Autodesk Inventor part; units mm, degrees
ref_plane "YZ Plane" through (0, 0, 0) normal (1, 0, 0) x (0, 1, 0)
ref_plane "XZ Plane" through (0, 0, 0) normal (0, 1, 0) x (-1, 0, 0)
ref_plane "XY Plane" through (0, 0, 0) normal (0, 0, 1) x (1, 0, 0)
sketch "Sketch1" plane through (0, 0, 0) normal (0, 1, 0) x (-1, 0, 0)
  line L0 (-5.5, -5.5) -> (-2, -5.5)
  line L1 (5.5, -0.5) -> (5.5, -0.5)
  line L2 (5.5, 5.5) -> (-5.5, 5.5)
  line L3 (-5.5, -0.5) -> (-5.5, -0.5)
  line L4 (-5.5, -5.5) -> (5.5, 5.5) construction
  line L5 (5.5, -5.5) -> (-5.5, 5.5) construction
  circle A0 centre (2.5, 2.5) radius 1
  circle A1 centre (-2.5, 2.5) radius 1
  line L6 (5.5, 5.5) -> (5.5, 2)
  line L7 (-5.5, 5.5) -> (-5.5, -5.5)
  circle A2 centre (-2.5, -2.5) radius 1
  arc A3 (-2, -5.5) -> (5.5, 2) centre (-2, 2) ccw
  point P0 (0, 0)
  dimension "d1" = 11
  dimension "d3" = 2
  dimension "d4" = 2
  dimension "d5" = 3
  dimension "d6" = 3
  dimension "d7" = 3
  dimension "d8" = 3
  dimension "d12" = 11
  dimension "d13" = 2
  dimension "d14" = 3
  dimension "d15" = 3
  dimension "d16" = 7.5
extrude "Extrusion1" add sketch "Sketch1" along normal blind 5
properties part number "link"
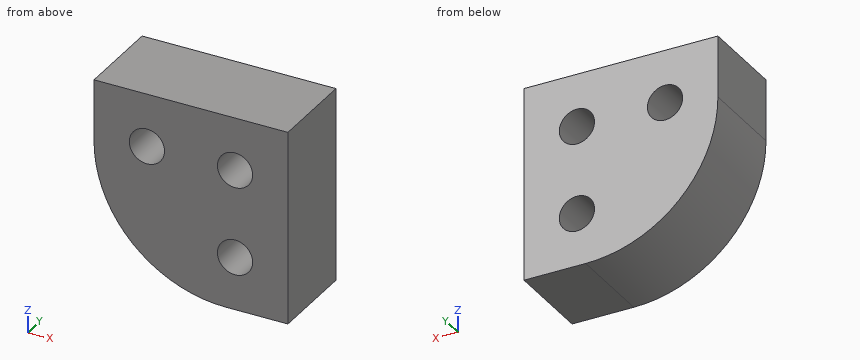
Geometry check sheet. Reference: the model listing, model coordinates, mm. Coordinates: 2 decimals unless noted, no trailing zeros. Order: outer loops, then holes, each group sorted by start corner. A loop starts at its lowest first (then second) coordinate and runs counter-clockwise, first axis right, second up.
Item 1: Section check A-A (z = -2.5). Enter the section's corners in (x, y).
Item 2: Section check D-D (y = 2.8). Enter the section's corners in (x, z).
Item 3: Section check B-B (x = -2.5). Enter the section's corners in (y, z), plus the area to 3 significant figures.
Item 4: Section check C-C (x = 2.5). Enter the section's corners in (y, z).
Item 5: Scan lines: line 1 along X through (y, z) = (2.5, 1.75); line 2 along Z through (x, y) = (-2.25, 4.2); line 3 along X through (y, z) = (3.15, 3). Record each from-to range of solid material in increasing order.
Check sheet entries:
1. outline: (-4, 0) - (1.5, 0) - (1.5, 5) - (-4, 5) - close; (3.5, 0) - (5.5, 0) - (5.5, 5) - (3.5, 5) - close
2. outline: (-5.5, 2) arc R7.5 ccw to (2, -5.5) - (5.5, -5.5) - (5.5, 5.5) - (-5.5, 5.5) - close; hole circle Ø2 at (-2.5, 2.5); hole circle Ø2 at (2.5, -2.5); hole circle Ø2 at (2.5, 2.5)
3. outline: (0, -4) - (5, -4) - (5, 1.5) - (0, 1.5) - close; (0, 3.5) - (5, 3.5) - (5, 5.5) - (0, 5.5) - close
3. area: 37.5 mm2
4. outline: (0, -5.5) - (5, -5.5) - (5, -3.5) - (0, -3.5) - close; (0, -1.5) - (5, -1.5) - (5, 1.5) - (0, 1.5) - close; (0, 3.5) - (5, 3.5) - (5, 5.5) - (0, 5.5) - close
5. line 1: x = -5.5 to -3.16, -1.84 to 1.84, 3.16 to 5.5
5. line 2: z = -4.18 to 1.53, 3.47 to 5.5
5. line 3: x = -5.5 to -3.37, -1.63 to 1.63, 3.37 to 5.5
